```python
from build123d import *

# Parameters (mm, degrees)
F0_W          = 7.6891479548
F0_H          = 6.0103421565
F1_DEPTH      = 10
F2_W          = 1.6820132732
F2_H          = 1.2127011675
F2_W_2        = 1.5973832924
F2_H_2        = 1.5515421644
F2_W_3        = 1.5004627639
F2_W_4        = 1.5929426299
F3_DEPTH      = 1.5
F4_R          = 1.7372427754
F5_DEPTH      = 25
F5_DEPTH_BACK = 25
F6_R          = 1.2262394043
F7_DEPTH      = 25
F7_DEPTH_BACK = 25
F8_R          = 1.7372427754
F9_DEPTH      = 2.5


with BuildPart() as f1:
    # F0 (on Top) → F1 (new body)
    with BuildSketch(Plane.XY):
        with Locations((-0.0009319047, 0.0121527119)):
            Rectangle(F0_W, F0_H)
    extrude(amount=F1_DEPTH)

    # F2 (on Top) → F3 (cut)
    with BuildSketch(Plane.XY):
        Polygon((-2.6183645241, 2.35), (-3.7, 2.35), (-3.7, -2.35), (-2.5337345432, -2.35), (-0.9363512509, -2.35), (1.0780681623, -2.35), (2.6710107923, -2.35), (3.7, -2.35), (3.7, 2.35), (2.6710107923, 2.35), (1.1705480283, 2.35), (-0.9363512509, 2.35), align=None)
        with Locations((-1.7773578875, 2.9563505838)):
            Rectangle(F2_W, F2_H)
        with Locations((-1.7350428971, -3.1257710822)):
            Rectangle(F2_W_2, F2_H_2)
        with Locations((1.9207794103, 2.9563505838)):
            Rectangle(F2_W_3, F2_H)
        with Locations((1.8745394773, -3.1257710822)):
            Rectangle(F2_W_4, F2_H_2)
    extrude(amount=F3_DEPTH, mode=Mode.SUBTRACT)

    # F4 (on Right) → F5 (cut, two sides)
    with BuildSketch(Plane.YZ) as f5_sk:
        with Locations((0, 4.3023279868)):
            Circle(F4_R)
    extrude(amount=-F5_DEPTH, mode=Mode.SUBTRACT)
    extrude(f5_sk.sketch, amount=F5_DEPTH_BACK, mode=Mode.SUBTRACT)

    # F6 (on Front) → F7 (cut, two sides)
    with BuildSketch(Plane.XZ) as f7_sk:
        with Locations((0, 7.6466021128)):
            Circle(F6_R)
    extrude(amount=F7_DEPTH, mode=Mode.SUBTRACT)
    extrude(f7_sk.sketch, amount=-F7_DEPTH_BACK, mode=Mode.SUBTRACT)

    # F8 (on face) → F9 (cut)
    with BuildSketch(Plane(origin=(-3.8455058821, 0, 0), x_dir=(0, -1, 0), z_dir=(-1, 0, 0))):
        Polygon((2.9930183664, 4.5848923734), (1.6247780807, 7.0305929156), (-1.5503576963, 7.0735595446), (-3.0173237901, 4.6102864409), (-3.0173237901, 4.0632090305), (-1.6247780807, 1.574063058), (1.5503576963, 1.531096429), (2.9930183664, 3.953556799), align=None)
        with Locations((0, 4.3023279868)):
            Circle(F8_R, mode=Mode.SUBTRACT)
    extrude(amount=-F9_DEPTH, mode=Mode.SUBTRACT)


solid = f1.part
```
Design review of the part built by this model. Coordinates are the model's own, in mm. A direction names the side the tool comes from. Round coordinates to 2 decimals unless told otherwise and drop trailing zeros. Write each loop counter-clockwise with the first axis right and the second up, starting at its lowest first coordinate (ties: lowest second). Pieces come first, ordered by that corner, then holes. Notation, with made-up numbers: (83.5, 1) -> (115.5, 1) arc R16 ccw to (115.5, 28) -> close; hole circle Ø1 at (62, 69). An arc over 180 degrees is marked (long way). Write item = value, one per line. Start each with the question number.
1) Mouldability with a two-part tool opening along Z and no side actions: class faces 4 (the face through (3, -2.35, 1)), 5 (the face through (-2.61, -2.32, 5.79)), 6 (the face through (1.285, -0.377, 2.606)) as +Z half, -Z half, draft (parallel to the pull), parting line (faces both ways), or undercut.
2) Tool access review of faces 1 (the face through (-2.613, 2.331, 2.836)), 2 (the face through (3, 2.35, 1)), 3 (the face through (3.844, -1, 6)): name each direction out of +Z, -Z, +X, -X, +Y, -Y from which nothing blocks a thin tool from reaching the whole face with its end or side.
3) Take a section at A-A, the plane x = -2.25. State the section outline as (y, z) points, plus the area to 3 significant figures.
4) Take a section at C-C, the plane x = 0.5. State the section outline as (y, z) points.
5) Wall thickness on probe 1 along Z at (x, y) = (0.05, 0); probe 2 along X at (y, z) = (2.75, 1); probe 3 along Z at (x, y) = (0, -1.5): over which ranges is each line inside the solid? List them lowest first. Write a range as from..to.
6) Take a section at B-B, the plane y = 0. State the section outline as (x, z) points.
7) Take a section at D-D, the plane z = 8.5. State the section outline as (x, y) points.
Results list:
q1.face_4 = draft
q1.face_5 = undercut
q1.face_6 = undercut
q2.face_1 = -X
q2.face_2 = -Z
q2.face_3 = +Z, -Z, +X, +Y, -Y
q3.outline = (-2.99, 1.5) -> (3.02, 1.5) -> (3.02, 4.06) -> (1.62, 1.57) -> (-1.55, 1.53) -> (-2.99, 3.95) -> close; (-2.99, 4.58) -> (-1.62, 7.03) -> (1.55, 7.07) -> (3.02, 4.61) -> (3.02, 10) -> (-2.99, 10) -> close
q3.area = 25.0 mm²
q4.outline = (-2.99, 0) -> (-2.35, 0) -> (-2.35, 1.5) -> (2.35, 1.5) -> (2.35, 0) -> (3.02, 0) -> (3.02, 6.53) -> (-2.99, 6.53) -> close; (-2.99, 8.77) -> (3.02, 8.77) -> (3.02, 10) -> (-2.99, 10) -> close; hole circle Ø3.47 at (0, 4.3)
q5.probe_1 = 1.5..2.57, 6.04..6.42, 8.87..10
q5.probe_2 = -3.85..-2.62, -0.94..1.17, 2.67..3.84
q5.probe_3 = 1.5..3.43, 5.18..6.42, 8.87..10
q6.outline = (-3.85, 0) -> (-3.7, 0) -> (-3.7, 1.5) -> (3.7, 1.5) -> (3.7, 0) -> (3.84, 0) -> (3.84, 2.57) -> (-1.35, 2.57) -> (-1.35, 1.55) -> (-3.85, 1.55) -> close; (-3.85, 7.05) -> (-1.35, 7.05) -> (-1.35, 6.04) -> (3.84, 6.04) -> (3.84, 10) -> (-3.85, 10) -> close; hole circle Ø2.45 at (0, 7.65)
q7.outline = (-3.85, -2.99) -> (-0.88, -2.99) -> (-0.88, 3.02) -> (-3.85, 3.02) -> close; (0.88, -2.99) -> (3.84, -2.99) -> (3.84, 3.02) -> (0.88, 3.02) -> close
